Could you check a few things on this model? Use its own coordinates, in mm. A direction names the side the tool comes from. Give positions to 0.01 mm unless a question says otherwise; leave off trailing zeros. Loops run counter-clockwise (first coordinate to the right, second up) from the corner with the lowest first, then second, coordinate; pieces in that order, holes last. Notation, with made-up numbers: (-6, 39) - (45, 39) arc R14 ccw to (45, 65) - close; hole circle Ø10 at (4, -3.5). An arc over 180 degrees is marked (long way). Use CSV: the item, a comma, the result in double quotes.
from build123d import *

# Parameters (mm, degrees)
SKETCH1_R                                       = 1.7
BOSS_EXTRUDE1_DEPTH                             = 2
BOSS_EXTRUDE2_DEPTH                             = 7.6
SKETCH3_W                                       = 2
SKETCH3_H                                       = 3
BOSS_EXTRUDE3_DEPTH                             = 4.5
CSK_FOR_M3_FLAT_HEAD_MACHINE_SCREW1_D           = 3.4
CSK_FOR_M3_FLAT_HEAD_MACHINE_SCREW1_CSINK_D     = 6.3
CSK_FOR_M3_FLAT_HEAD_MACHINE_SCREW1_CSINK_ANGLE = 90
SKETCH6_W                                       = 2
SKETCH6_H                                       = 8.265
SKETCH6_H_2                                     = 8.335
SKETCH6_H_3                                     = 3.6
CUT_EXTRUDE1_DEPTH                              = 1
GROOVE2_START                                   = -18
GROOVE2_OUTLINE_W                               = 58
GROOVE2_OUTLINE_H                               = 2
GROOVE2_DEPTH                                   = 36.20069
GROOVE2_START_2                                 = 7.697541275
GROOVE2_2_DEPTH                                 = 8.902458725
GROOVE2_START_3                                 = -16.6
GROOVE2_3_DEPTH                                 = 9.9
GROOVE2_START_4                                 = 1.5
GROOVE2_4_DEPTH                                 = 6.197541275
GROOVE2_5_DEPTH                                 = 4.697541275
BOSS_EXTRUDE4_DEPTH                             = 1


with BuildPart() as part:
    # Sketch1 → Boss-Extrude1 (new body)
    with BuildSketch(Plane(origin=(0, 0, 0), x_dir=(1, 0, 0), z_dir=(0, 1, 0))):
        with BuildLine():
            Line((-27.6, 20), (27.6, 20))
            ThreePointArc((27.6, 20), (30.004163056, 19.004163056), (31, 16.6))
            Line((31, 16.6), (31, -16.6))
            ThreePointArc((31, -16.6), (30.004163056, -19.004163056), (27.6, -20))
            Line((27.6, -20), (-27.6, -20))
            ThreePointArc((-27.6, -20), (-30.004163056, -19.004163056), (-31, -16.6))
            Line((-31, -16.6), (-31, 16.6))
            ThreePointArc((-31, 16.6), (-30.004163056, 19.004163056), (-27.6, 20))
        make_face()
        with Locations(Location((-25, -12.06, 0), (0, 0, 270))):
            Circle(SKETCH1_R, mode=Mode.SUBTRACT)
        with Locations(Location((25, -12.06, 0), (0, 0, 270))):
            Circle(SKETCH1_R, mode=Mode.SUBTRACT)
        with Locations(Location((25, 12.94, 0), (0, 0, 270))):
            Circle(SKETCH1_R, mode=Mode.SUBTRACT)
    extrude(amount=BOSS_EXTRUDE1_DEPTH)

    # Sketch2 → Boss-Extrude2 (add)
    with BuildSketch(Plane(origin=(0, 2, 0), x_dir=(1, 0, 0), z_dir=(0, 1, 0))):
        with BuildLine():
            Line((-27.6, -20), (27.6, -20))
            ThreePointArc((27.6, -20), (30.004163056, -19.004163056), (31, -16.6))
            Line((31, -16.6), (31, 16.6))
            ThreePointArc((31, 16.6), (30.004163056, 19.004163056), (27.6, 20))
            Line((27.6, 20), (-27.6, 20))
            ThreePointArc((-27.6, 20), (-30.004163056, 19.004163056), (-31, 16.6))
            Line((-31, 16.6), (-31, -16.6))
            ThreePointArc((-31, -16.6), (-30.004163056, -19.004163056), (-27.6, -20))
        make_face()
        with BuildLine():
            Line((27.6, 18), (-27.6, 18))
            ThreePointArc((-27.6, 18), (-28.589949494, 17.589949494), (-29, 16.6))
            Line((-29, 16.6), (-29, -16.6))
            ThreePointArc((-29, -16.6), (-28.589949494, -17.589949494), (-27.6, -18))
            Line((-27.6, -18), (27.6, -18))
            ThreePointArc((27.6, -18), (28.589949494, -17.589949494), (29, -16.6))
            Line((29, -16.6), (29, 16.6))
            ThreePointArc((29, 16.6), (28.589949494, 17.589949494), (27.6, 18))
        make_face(mode=Mode.SUBTRACT)
    extrude(amount=BOSS_EXTRUDE2_DEPTH)

    # Sketch3 → Boss-Extrude3 (add)
    with BuildSketch(Plane(origin=(0, 9.6, 0), x_dir=(1, 0, 0), z_dir=(0, 1, 0))):
        with Locations((-30, 2.137458725)):
            Rectangle(SKETCH3_W, SKETCH3_H)
    extrude(amount=BOSS_EXTRUDE3_DEPTH)

    # CSK for M3 Flat Head Machine Screw1 (through all)
    with Locations(Plane(origin=(-25, 0, 12.06), x_dir=(0, 0, -1), z_dir=(0, -1, 0))):
        with Locations((0, 0), (0, 50), (25, 50)):
            CounterSinkHole(CSK_FOR_M3_FLAT_HEAD_MACHINE_SCREW1_D / 2, CSK_FOR_M3_FLAT_HEAD_MACHINE_SCREW1_CSINK_D / 2, counter_sink_angle=CSK_FOR_M3_FLAT_HEAD_MACHINE_SCREW1_CSINK_ANGLE)

    # Sketch6 → Cut-Extrude1 (cut)
    with BuildSketch(Plane(origin=(0, 9.6, 0), x_dir=(1, 0, 0), z_dir=(0, 1, 0))):
        with Locations((-30, 7.769958725)):
            Rectangle(SKETCH6_W, SKETCH6_H)
        with Locations((-30, -3.530041275)):
            Rectangle(SKETCH6_W, SKETCH6_H_2)
        with Locations((30, 4.9)):
            Rectangle(SKETCH6_W, SKETCH6_H_3)
        with Locations((30, 0.3)):
            Rectangle(SKETCH6_W, SKETCH6_H_3)
    extrude(amount=-CUT_EXTRUDE1_DEPTH, mode=Mode.SUBTRACT)

    # Groove2: read off the stored shape, not the designer's step
    # Groove2 outline → Groove2 (cut)
    with BuildSketch(Plane.XY.offset(GROOVE2_START)):
        with Locations((0, 8.6)):
            Rectangle(GROOVE2_OUTLINE_W, GROOVE2_OUTLINE_H)
    extrude(amount=GROOVE2_DEPTH, mode=Mode.SUBTRACT)

    # Groove2 2 outline → Groove2 2 (cut)
    with BuildSketch(Plane.XY.offset(GROOVE2_START_2)):
        Polygon((29, 7.6), (29.895184441, 7.6), (30, 9.6), (29, 9.6), align=None)
        Polygon((-29.895184441, 7.6), (-29, 7.6), (-29, 9.6), (-30, 9.6), align=None)
    extrude(amount=GROOVE2_2_DEPTH, mode=Mode.SUBTRACT)

    # Groove2 3 outline → Groove2 3 (cut)
    with BuildSketch(Plane.XY.offset(GROOVE2_START_3)):
        Polygon((29, 7.6), (29.895184441, 7.6), (30, 9.6), (29, 9.6), align=None)
    extrude(amount=GROOVE2_3_DEPTH, mode=Mode.SUBTRACT)

    # Groove2 4 outline → Groove2 4 (cut)
    with BuildSketch(Plane.XY.offset(GROOVE2_START_4)):
        Polygon((29, 7.6), (29.895184441, 7.6), (30, 9.6), (29, 9.6), align=None)
    extrude(amount=GROOVE2_4_DEPTH, mode=Mode.SUBTRACT)

    # Groove2 5 outline → Groove2 5 (cut)
    with BuildSketch(Plane.XY.offset(GROOVE2_START_3)):
        Polygon((-29.895184441, 7.6), (-29, 7.6), (-29, 9.6), (-30, 9.6), align=None)
    extrude(amount=GROOVE2_5_DEPTH, mode=Mode.SUBTRACT)

    # Groove2 6: loft between two sections, ruled curve by curve
    groove2_6_from = [
        Edge.make_three_point_arc((-29.895184441, 7.6, 16.6), (-29.222940483, 7.6, 18.222940483), (-27.6, 7.6, 18.895184441)),
        Edge.make_three_point_arc((27.6, 7.6, 18.895184441), (29.222940483, 7.6, 18.222940483), (29.895184441, 7.6, 16.6)),
        Edge.make_line((27.6, 7.6, 18.895184441), (-27.6, 7.6, 18.895184441)),
        Edge.make_line((29.895184441, 7.6, 16.6), (-29.895184441, 7.6, 16.6)),
    ]
    groove2_6_to = [
        Edge.make_three_point_arc((-30, 9.6, 16.6), (-29.297056275, 9.6, 18.297056275), (-27.6, 9.6, 19)),
        Edge.make_three_point_arc((27.6, 9.6, 19), (29.297056275, 9.6, 18.297056275), (30, 9.6, 16.6)),
        Edge.make_line((27.6, 9.6, 19), (-27.6, 9.6, 19)),
        Edge.make_line((30, 9.6, 16.6), (-30, 9.6, 16.6)),
    ]
    groove2_6 = Solid(Shell([*[Face.make_surface_from_curves(groove2_6_from[k], groove2_6_to[k]) for k in range(4)], Face(Wire(groove2_6_from)), Face(Wire(groove2_6_to))]))
    add(groove2_6, mode=Mode.SUBTRACT)

    # Groove2 7: loft between two sections, ruled curve by curve
    groove2_7_from = [
        Edge.make_three_point_arc((29.895184441, 7.6, -16.6), (29.222940483, 7.6, -18.222940483), (27.6, 7.6, -18.895184441)),
        Edge.make_three_point_arc((-27.6, 7.6, -18.895184441), (-29.222940483, 7.6, -18.222940483), (-29.895184441, 7.6, -16.6)),
        Edge.make_line((-27.6, 7.6, -18.895184441), (27.6, 7.6, -18.895184441)),
        Edge.make_line((-29.895184441, 7.6, -16.6), (29.895184441, 7.6, -16.6)),
    ]
    groove2_7_to = [
        Edge.make_three_point_arc((30, 9.6, -16.6), (29.297056275, 9.6, -18.297056275), (27.6, 9.6, -19)),
        Edge.make_three_point_arc((-27.6, 9.6, -19), (-29.297056275, 9.6, -18.297056275), (-30, 9.6, -16.6)),
        Edge.make_line((-27.6, 9.6, -19), (27.6, 9.6, -19)),
        Edge.make_line((-30, 9.6, -16.6), (30, 9.6, -16.6)),
    ]
    groove2_7 = Solid(Shell([*[Face.make_surface_from_curves(groove2_7_from[k], groove2_7_to[k]) for k in range(4)], Face(Wire(groove2_7_from)), Face(Wire(groove2_7_to))]))
    add(groove2_7, mode=Mode.SUBTRACT)

    # Sketch7 → Boss-Extrude4 (add)
    with BuildSketch(Plane(origin=(0, 8.6, 0), x_dir=(1, 0, 0), z_dir=(0, 1, 0))):
        Polygon((-31, 11.902458725), (-31, 3.637458725), (-29, 3.637458725), (-29, 11.902458725), (-29.947592221, 11.902458725), align=None)
        Polygon((-29, -7.697541275), (-29, 0.637458725), (-31, 0.637458725), (-31, -7.697541275), (-29.947592221, -7.697541275), align=None)
        Polygon((29, 3.1), (31, 3.1), (31, 6.7), (29.947592221, 6.7), (29, 6.7), align=None)
        Polygon((31, 2.1), (29, 2.1), (29, -1.5), (29.947592221, -1.5), (31, -1.5), align=None)
    extrude(amount=BOSS_EXTRUDE4_DEPTH)


solid = part.part
1) Suppose I cut it at D-D (x = 25). State how many separate pieces and enclosed holes the cut face has, plus the area to 3 significant figures.
Answer below:
separate pieces,"3"
enclosed holes,"0"
area,"88.8 mm2"
2) Suppose I cut it at B-B (y = 6). Please give me the cut outline in (x, z).
Answer below:
outline,"(-31, -16.6) arc R3.4 ccw to (-27.6, -20) - (27.6, -20) arc R3.4 ccw to (31, -16.6) - (31, 16.6) arc R3.4 ccw to (27.6, 20) - (-27.6, 20) arc R3.4 ccw to (-31, 16.6) - close; hole (-29, -16.6) arc R1.4 ccw to (-27.6, -18) - (27.6, -18) arc R1.4 ccw to (29, -16.6) - (29, 16.6) arc R1.4 ccw to (27.6, 18) - (-27.6, 18) arc R1.4 ccw to (-29, 16.6) - close"
3) I need wall thicknesses on line 1 along Z through (x, y) = (25, 1.85); line 2 along X through (y, z) = (1.7, 12.06); line 3 along X through (y, z) = (7, -6.5). Which ranges of each line are inside material? Lowest first, please.
Answer below:
line 1,"z = -20 to -14.64, -11.24 to 10.36, 13.76 to 20"
line 2,"x = -31 to -26.7, -23.3 to 23.3, 26.7 to 31"
line 3,"x = -31 to -29, 29 to 31"
4) We'd pull the mould along Z, two halves only. Please class faces 1 (the flat face through (0, 5, -20)), 2 (the flat face through (-0.1, 7.6, 18.5)), 3 (the cylindrical face through (29.98, 4.73, 19.03)): +Z half, -Z half, draft (parallel to the pull), parting line (faces both ways), or undercut.
Answer below:
face 1,"-Z half"
face 2,"undercut"
face 3,"+Z half"
5) Suppose I cut it at A-A (z = -12.94). Please give me the cut outline in (x, y).
Answer below:
outline,"(-31, 0) - (21.85, 0) - (23.3, 1.45) - (23.3, 2) - (-29, 2) - (-29, 7.6) - (-29.9, 7.6) - (-30, 9.6) - (-31, 9.6) - close; (26.7, 1.45) - (28.15, 0) - (31, 0) - (31, 9.6) - (30, 9.6) - (29.9, 7.6) - (29, 7.6) - (29, 2) - (26.7, 2) - close"
6) I'm going to push flat-ended pins straight in: P1, Ø6, axis at x = 12.5, z = -14, coming from the +Y side; P2, Ø4, axis at x = -25, z = 12.06, coming from the -Y side; P3, Ø1.1, axis at x = -29.5, y = 8.5, coming from the -Z side. Where does each tip first touch, or does it pass through?
Answer below:
P1,"stops at y = 2"
P2,"stops at y = 1.15"
P3,"stops at z = -19.72"
7) Which directions (+Z, -Z, +X, -X, +Y, -Y) give clear straight access to the entire face, cutting with the end or side of a thin tool? Please do faces 4 (the flat face through (-29, 7, 0)), 5 (the cylindrical face through (30.03, 4.73, -18.98)).
Answer below:
face 4,"+Y"
face 5,"-Z, +X, +Y, -Y"
8) Suppose I cut it at C-C (z = 12.06). Please give me the cut outline in (x, y).
Answer below:
outline,"(-31, 0) - (-28.15, 0) - (-26.7, 1.45) - (-26.7, 2) - (-29, 2) - (-29, 7.6) - (-29.9, 7.6) - (-30, 9.6) - (-31, 9.6) - close; (-23.3, 1.45) - (-21.85, 0) - (21.85, 0) - (23.3, 1.45) - (23.3, 2) - (-23.3, 2) - close; (26.7, 1.45) - (28.15, 0) - (31, 0) - (31, 9.6) - (30, 9.6) - (29.9, 7.6) - (29, 7.6) - (29, 2) - (26.7, 2) - close"
